from build123d import *

# Parameters (mm, degrees)
BASE_EXTRUDE_THIN_DEPTH = 20
CUT_EXTRUDE1_REACH      = 187.74
SKETCH2_R               = 6.25
CUT_EXTRUDE2_REACH      = 207
SKETCH3_R               = 6.25


with BuildPart() as part:
    # Sketch1 → Base-Extrude-Thin (new, symmetric)
    with BuildSketch(Plane.XY):
        with BuildLine():
            Line((0, 120), (0, 5))
            ThreePointArc((0, 5), (1.464466094, 1.464466094), (5, 0))
            Line((5, 0), (145, 0))
            ThreePointArc((145, 0), (148.535533906, 1.464466094), (150, 5))
            Line((150, 5), (150, 55))
            Line((150, 55), (157.5, 55))
            Line((157.5, 55), (157.5, 5))
            ThreePointArc((157.5, 5), (153.838834765, -3.838834765), (145, -7.5))
            Line((145, -7.5), (5, -7.5))
            ThreePointArc((5, -7.5), (-3.838834765, -3.838834765), (-7.5, 5))
            Line((-7.5, 5), (-7.5, 120))
            Line((-7.5, 120), (0, 120))
        make_face()
    extrude(amount=BASE_EXTRUDE_THIN_DEPTH, both=True)

    # Sketch2 → Cut-Extrude1 (cut, up to next)
    with BuildSketch(Plane(origin=(0, 88.9, 0), x_dir=(0, -1, 0), z_dir=(-1, 0, 0)), mode=Mode.PRIVATE) as cut_extrude1_sk1:
        with Locations(Location((-16.1, 0, 0), (0, 0, 270))):
            Circle(SKETCH2_R)
    cut_extrude1_tool1 = extrude(cut_extrude1_sk1.sketch, amount=CUT_EXTRUDE1_REACH, mode=Mode.PRIVATE) & part.part
    add(cut_extrude1_tool1.solids().sort_by_distance((0, 105, 0))[0], mode=Mode.SUBTRACT)

    # Sketch3 → Cut-Extrude2 (cut, up to next)
    with BuildSketch(Plane(origin=(157.5, 0, 0), x_dir=(0, 0, -1), z_dir=(1, 0, 0)), mode=Mode.PRIVATE) as cut_extrude2_sk1:
        with Locations(Location((0, 40, 0), (0, 0, 90))):
            Circle(SKETCH3_R)
    cut_extrude2_tool1 = extrude(cut_extrude2_sk1.sketch, amount=-CUT_EXTRUDE2_REACH, mode=Mode.PRIVATE) & part.part
    add(cut_extrude2_tool1.solids().sort_by_distance((157.5, 40, 0))[0], mode=Mode.SUBTRACT)


solid = part.part
CAD build for the part. Positions are in the model's coordinates, mm. A direction names the side the tool comes from. Round coordinates to 2 decimals unless told otherwise and drop trailing zeros. Write each loop counter-clockwise with the first axis right and the second up, starting at its lowest first coordinate (ties: lowest second). Pieces come first, ordered by that corner, then holes. Notation, with made-up numbers: M 59.25,83 L 106.25,83 A25 cw 106.25,114 Z; hole C 55.25,-38 d6. An arc over 180 degrees is marked long. Use a Markdown table: item, result. Add a question column.
1. Drill centre lines: probe 1 along X at (y, z) = (35, -14.5); probe 2 along Z at (x, y) = (152, 40); probe 3 along X at (y, z) = (85, -2). Where is each one in solid material? Low to high.
2. Slice it at A-A on z = 0. Give the cut face in (x, y), then the cut area to 3 significant figures.
3. 3-axis set-ups, long thin cutter, end or side, ignore diameter. For faces 4 (the face through (-3.7, 98.8, 0.8)), 5 (the face through (-3.741, -3.935, 0.28)), 6 (the face through (154, 55, 0)), 7 (the face through (153.8, 45.96, 1.88)), 8 (the face through (150, 30, 0)): which of +Z, -Z, +X, -X, +Y, -Y reach the whole face in a straight line?
4. Slice it at B-B on y = 105. Give the cut face in (x, z).
5. Flat gauge pins, fed straight in: P1, Ø7.5, axis at y = 105, z = 0, coming from the -X side; P2, Ø5, axis at x = 100, z = 1, coming from the +Y side; P3, Ø2, axis at x = 154, z = -1, coming from the +Y side; P4, Ø8, axis at y = 79, z = 0.5, coming from the +X side. Where does each tip first touch, or does it go through?
6. Slice it at C-C on y = 40. Give the cut face in (x, z).
7. Pull direction X, two halves, no side cores. Call faces 1 (the face through (74, 0, 0)), 2 (the face through (-7.5, 62, 0)), 3 (the face through (157.5, 30, 0)): released by +X, released by -X, zero draft, split by the parting line, or undercut.
8. Slice it at D-D on z = 9.5. Give the cut face in (x, y), then the cut area to 3 significant figures.
Reply:
| question | item | result |
|---|---|---|
| 1 | probe 1 | x = -7.5 to 0, 150 to 157.5 |
| 1 | probe 2 | z = -20 to -6.25, 6.25 to 20 |
| 1 | probe 3 | x = -7.5 to 0 |
| 2 | outline | M -7.5,5 A12.5 ccw 5,-7.5 L 145,-7.5 A12.5 ccw 157.5,5 L 157.5,33.75 L 150,33.75 L 150,5 A5 cw 145,0 L 5,0 A5 cw 0,5 L 0,98.75 L -7.5,98.75 Z; M -7.5,111.25 L 0,111.25 L 0,120 L -7.5,120 Z; M 150,46.25 L 157.5,46.25 L 157.5,55 L 150,55 Z |
| 2 | area | 2,310 mm^2 |
| 3 | face 4 | +X, -X |
| 3 | face 5 | +Z, -Z, -X, -Y |
| 3 | face 6 | +Z, -Z, +X, +Y |
| 3 | face 7 | +X |
| 3 | face 8 | +Z, -Z, +Y |
| 4 | outline | M -7.5,-20 L 0,-20 L 0,-6.25 L -7.5,-6.25 Z; M -7.5,6.25 L 0,6.25 L 0,20 L -7.5,20 Z |
| 5 | P1 | passes through |
| 5 | P2 | stops at y = 0 |
| 5 | P3 | stops at y = 55 |
| 5 | P4 | stops at x = 0 |
| 6 | outline | M -7.5,-20 L 0,-20 L 0,20 L -7.5,20 Z; M 150,-20 L 157.5,-20 L 157.5,-6.25 L 150,-6.25 Z; M 150,6.25 L 157.5,6.25 L 157.5,20 L 150,20 Z |
| 7 | face 1 | undercut |
| 7 | face 2 | released by -X |
| 7 | face 3 | released by +X |
| 8 | outline | M -7.5,5 A12.5 ccw 5,-7.5 L 145,-7.5 A12.5 ccw 157.5,5 L 157.5,55 L 150,55 L 150,5 A5 cw 145,0 L 5,0 A5 cw 0,5 L 0,120 L -7.5,120 Z |
| 8 | area | 2,490 mm^2 |
